```python
from build123d import *

# Parameters (mm, degrees)
SKETCH_1_W                  = 86
SKETCH_1_H                  = 44.2
EXTRUDE_1_DEPTH             = 14.2
EXTRUDE_2_DEPTH             = 5
SKETCH_3_W                  = 26.584
SKETCH_3_H                  = 42.4
CUT_EXTRUDE_1_DEPTH         = 18.3
SKETCH_4_W                  = 26.583
SKETCH_4_H                  = 42.4
CUT_EXTRUDE_2_DEPTH         = 18.3
SKETCH_5_W                  = 26.133
SKETCH_5_H                  = 42.4
CUT_EXTRUDE_3_DEPTH         = 18.3
HOLE_WIZARD_8_3_8_3_1_D     = 8.3
HOLE_WIZARD_8_3_8_3_1_DEPTH = 3.2
HOLE_WIZARD_6_0_6_1_D       = 6
HOLE_WIZARD_6_0_6_1_DEPTH   = 0.9
HOLE_WIZARD_6_0_6_2_D       = 6
HOLE_WIZARD_6_0_6_2_DEPTH   = 0.9
FILLET_1_R                  = 3
EXTRUDE_START               = -3.5
SKETCH_12_R                 = 4.15
EXTRUDE_3_DEPTH             = 3.5
FILLET_2_R                  = 2


with BuildPart() as part:
    # Эскиз1 → Бобышка-Вытянуть1 (new body)
    with BuildSketch(Plane.XY.offset(9.6)):
        with Locations((47, 0)):
            Rectangle(SKETCH_1_W, SKETCH_1_H)
    extrude(amount=-EXTRUDE_1_DEPTH)

    # Эскиз2 → Бобышка-Вытянуть2 (add)
    with BuildSketch(Plane(origin=(0, 0, -4.6), x_dir=(-1, 0, 0), z_dir=(0, 0, -1))):
        with BuildLine():
            Line((-90, -22.1), (-90, -17.1))
            ThreePointArc((-90, -17.1), (-104, 0), (-90, 17.1))
            Line((-90, 17.1), (-90, 22.1))
            Line((-90, 22.1), (-4, 22.1))
            Line((-4, 22.1), (-4, -22.1))
            Line((-4, -22.1), (-90, -22.1))
        make_face()
        with BuildLine():
            Line((-90, -12.994779171), (-90, 12.994779171))
            ThreePointArc((-90, 12.994779171), (-100, 0), (-90, -12.994779171))
        make_face(mode=Mode.SUBTRACT)
    extrude(amount=EXTRUDE_2_DEPTH)

    # Эскиз3 → Вырез-Вытянуть1 (cut)
    with BuildSketch(Plane.XY.offset(9.6)):
        with Locations((75.808, 0)):
            Rectangle(SKETCH_3_W, SKETCH_3_H)
    extrude(amount=-CUT_EXTRUDE_1_DEPTH, mode=Mode.SUBTRACT)

    # Эскиз4 → Вырез-Вытянуть2 (cut)
    with BuildSketch(Plane.XY.offset(9.6)):
        with Locations((21.2915, 0)):
            Rectangle(SKETCH_4_W, SKETCH_4_H)
    extrude(amount=-CUT_EXTRUDE_2_DEPTH, mode=Mode.SUBTRACT)

    # Эскиз5 → Вырез-Вытянуть3 (cut)
    with BuildSketch(Plane.XY.offset(9.6)):
        with Locations((48.5495, 0)):
            Rectangle(SKETCH_5_W, SKETCH_5_H)
    extrude(amount=-CUT_EXTRUDE_3_DEPTH, mode=Mode.SUBTRACT)

    # Диаметр отверстия Ø8.3 (8.3)1
    with Locations(Plane.ZY.offset(-4)):
        with Locations((0, 0)):
            Hole(HOLE_WIZARD_8_3_8_3_1_D / 2, depth=HOLE_WIZARD_8_3_8_3_1_DEPTH)

    # Диаметр отверстия Ø6.0 (6)1
    with Locations(Plane.ZY.offset(-61.616)):
        with Locations((9.6, 0)):
            Hole(HOLE_WIZARD_6_0_6_1_D / 2, depth=HOLE_WIZARD_6_0_6_1_DEPTH)

    # Диаметр отверстия Ø6.0 (6)2
    with Locations(Plane(origin=(35.483, 0, 0), x_dir=(0, 0, -1), z_dir=(1, 0, 0))):
        with Locations((-9.6, 0)):
            Hole(HOLE_WIZARD_6_0_6_2_D / 2, depth=HOLE_WIZARD_6_0_6_2_DEPTH)

    # Скругление1
    fillet_1_edges = [part.edges().sort_by_distance(p)[0] for p in [
        (4, -22.1, 0),
        (4, 22.1, 0),
    ]]
    fillet(fillet_1_edges, radius=FILLET_1_R)

    # Эскиз12 → Бобышка-Вытянуть3 (add)
    with BuildSketch(Plane.ZY.offset(-4).offset(EXTRUDE_START)):
        Circle(SKETCH_12_R)
    extrude(amount=EXTRUDE_3_DEPTH)

    # Скругление2
    fillet_2_edges = [part.edges().sort_by_distance(p)[0] for p in [
        (90, -15.047389586, -4.6),
        (90, 15.047389586, -4.6),
        (75.808, 21.2, -8.7),
        (62.516, 21.2, 0.45),
        (89.1, 0, -8.7),
        (89.1, 21.2, 0.45),
        (75.808, -21.2, -8.7),
        (89.1, -21.2, 0.45),
        (62.516, 0, -8.7),
        (62.516, -21.2, 0.45),
        (21.2915, 21.2, -8.7),
        (8, 21.2, 0.45),
        (34.583, 0, -8.7),
        (34.583, 21.2, 0.45),
        (21.2915, -21.2, -8.7),
        (34.583, -21.2, 0.45),
        (8, 0, -8.7),
        (8, -21.2, 0.45),
        (48.5495, -21.2, -8.7),
        (61.616, -21.2, 0.45),
        (35.483, 0, -8.7),
        (35.483, -21.2, 0.45),
        (48.5495, 21.2, -8.7),
        (35.483, 21.2, 0.45),
        (61.616, 0, -8.7),
        (61.616, 21.2, 0.45),
    ]]
    fillet(fillet_2_edges, radius=FILLET_2_R)


solid = part.part
```
Geometry check sheet. Reference: the model listing, model coordinates, mm. Round coordinates to 2 decimals unless told otherwise and drop trailing zeros. Order: outer loops, then holes, each group sorted by start corner. A loop starts at its lowest first (then second) coordinate and runs counter-clockwise, first axis right, second up. Notation, with made-up numbers: M 51,75 L 74,75 A16 ccw 74,99 Z; hole C 15,53.25 d1. An arc over 180 degrees is marked long. Write item = value, one per line.
Q1. Scan lines: line 1 (X direction, y = 18.5, z = 2); line 2 (Y direction, x = 24, z = 0.25); line 3 (X direction, y = -16, z = -6.25). Record each from-to range of solid material in increasing order.
Answer block:
line_1 = 4 to 8, 34.58 to 35.48, 61.62 to 62.52, 89.1 to 90
line_2 = -22.1 to -21.2, 21.2 to 22.1
line_3 = 4 to 8, 34.58 to 35.48, 61.62 to 62.52, 89.1 to 93.5
Q2. Release check for a two-part mould opening along Y. For faces 1 (the flat face through (48, 22.1, 0)), 2 (the flat face through (76, 0, -8.7)), 3 (the flat face through (27.7, 21.4, 9.6)) record: released by +Y, released by -Y, zero draft, split by the parting line, or undercut.
Answer block:
face_1 = released by +Y
face_2 = undercut
face_3 = zero draft
Q3. Section check B-B (z = 4.5). Give the number of separate pieces and of enclosed holes in the cut face, plus the area to 3 significant figures.
Answer block:
separate_pieces = 1
enclosed_holes = 3
area = 445 mm^2
Q4. Depth check by flat-ended pin: pin 1 Ø6 at (y, z) = (14.5, 6) entering from +X; pin 2 Ø8 at (y, z) = (11, -5) entering from +X; pin 3 Ø9.5 at (x, y) = (98, 8) entering from +Z. Enter the tip coordinate at first touch or a pass-through.
Answer block:
pin_1 = 90
pin_2 = 102.53
pin_3 = -4.6
Q5. Section check A-A (y = 0). Enter the section's corners in (x, z).
Answer block:
outline = M 4,-9.6 L 90,-9.6 L 90,9.6 L 89.1,9.6 L 89.1,-6.7 A2 cw 87.1,-8.7 L 64.52,-8.7 A2 cw 62.52,-6.7 L 62.52,6.6 L 61.62,6.6 L 61.62,-6.7 A2 cw 59.62,-8.7 L 37.48,-8.7 A2 cw 35.48,-6.7 L 35.48,6.6 L 34.58,6.6 L 34.58,-6.7 A2 cw 32.58,-8.7 L 10,-8.7 A2 cw 8,-6.7 L 8,9.6 L 4,9.6 Z; M 100,-9.6 L 104,-9.6 L 104,-4.6 L 100,-4.6 Z
Q6. Section check D-D (y = 15). Enter the section's corners in (x, z), plus the area to 3 significant figures.
Answer block:
outline = M 4,-9.6 L 95.46,-9.6 L 95.46,-4.6 L 92,-4.6 A2 cw 90,-2.6 L 90,9.6 L 89.1,9.6 L 89.1,-6.7 A2 cw 87.1,-8.7 L 64.52,-8.7 A2 cw 62.52,-6.7 L 62.52,9.6 L 61.62,9.6 L 61.62,-6.7 A2 cw 59.62,-8.7 L 37.48,-8.7 A2 cw 35.48,-6.7 L 35.48,9.6 L 34.58,9.6 L 34.58,-6.7 A2 cw 32.58,-8.7 L 10,-8.7 A2 cw 8,-6.7 L 8,9.6 L 4,9.6 Z
area = 233 mm^2
Q7. Section check C-C (x = 70). Enter the section's corners in (y, z).
Answer block:
outline = M -22.1,-9.6 L 22.1,-9.6 L 22.1,9.6 L 21.2,9.6 L 21.2,-6.7 A2 cw 19.2,-8.7 L -19.2,-8.7 A2 cw -21.2,-6.7 L -21.2,9.6 L -22.1,9.6 Z
